```python
from build123d import *

# Parameters (mm, degrees)
BOSS_EXTRUDE1_DEPTH = 1.5875
SKETCH3_R           = 2.032
SKETCH3_R_2         = 1.778
CUT_EXTRUDE1_DEPTH  = 52.085937461
CUT_EXTRUDE2_DEPTH  = 52.085937461
FILLET1_R           = 6.35
FILLET2_R           = 1.5875


with BuildPart() as part:
    # Sketch1 → Boss-Extrude1 (new body)
    with BuildSketch(Plane(origin=(0, 0, 0), x_dir=(1, 0, 0), z_dir=(0, 1, 0))):
        with BuildLine():
            Line((0, 0), (18.415, -19.05))
            Line((18.415, -19.05), (18.415, -47.625))
            ThreePointArc((18.415, -47.625), (0, -46.266231115), (-18.415, -47.625))
            Line((-18.415, -47.625), (-18.415, -19.05))
            Line((-18.415, -19.05), (0, 0))
        make_face()
    extrude(amount=BOSS_EXTRUDE1_DEPTH)

    # Sketch3 → Cut-Extrude1 (cut, through all)
    with BuildSketch(Plane(origin=(0, 1.5875, 0), x_dir=(1, 0, 0), z_dir=(0, 1, 0))):
        with Locations(Location((12.7, -42.294109534, 0), (0, 0, 270))):
            Circle(SKETCH3_R)
        with Locations(Location((-12.7, -42.294109534, 0), (0, 0, 270))):
            Circle(SKETCH3_R)
        with Locations(Location((-12.7, -23.244109534, 0), (0, 0, 270))):
            Circle(SKETCH3_R)
        with Locations(Location((12.7, -23.244109534, 0), (0, 0, 270))):
            Circle(SKETCH3_R_2)
        with Locations(Location((0, -7.9375, 0), (0, 0, 270))):
            Circle(SKETCH3_R)
    extrude(amount=-CUT_EXTRUDE1_DEPTH, mode=Mode.SUBTRACT)

    # Sketch4 → Cut-Extrude2 (cut, through all)
    with BuildSketch(Plane(origin=(0, 1.5875, 0), x_dir=(1, 0, 0), z_dir=(0, 1, 0))):
        with BuildLine():
            Line((7.9375, -36.974796609), (7.9375, -23.286267168))
            Line((7.9375, -23.286267168), (0, -15.075060272))
            Line((0, -15.075060272), (-7.9375, -23.286267168))
            Line((-7.9375, -23.286267168), (-7.9375, -36.974796609))
            ThreePointArc((-7.9375, -36.974796609), (0, -36.741231115), (7.9375, -36.974796609))
        make_face()
    extrude(amount=-CUT_EXTRUDE2_DEPTH, mode=Mode.SUBTRACT)

    # Fillet1
    fillet1_edges = [part.edges().sort_by_distance(p)[0] for p in [
        (0, 0.79375, 0),
        (18.415, 0.79375, 19.05),
        (18.415, 0.79375, 47.625),
        (-18.415, 0.79375, 47.625),
        (-18.415, 0.79375, 19.05),
    ]]
    fillet(fillet1_edges, radius=FILLET1_R)

    # Fillet2
    fillet2_edges = [part.edges().sort_by_distance(p)[0] for p in [
        (-7.9375, 0.79375, 23.286267168),
        (0, 0.79375, 15.075060272),
        (7.9375, 0.79375, 23.286267168),
        (7.9375, 0.79375, 36.974796609),
        (-7.9375, 0.79375, 36.974796609),
    ]]
    fillet(fillet2_edges, radius=FILLET2_R)


solid = part.part
```
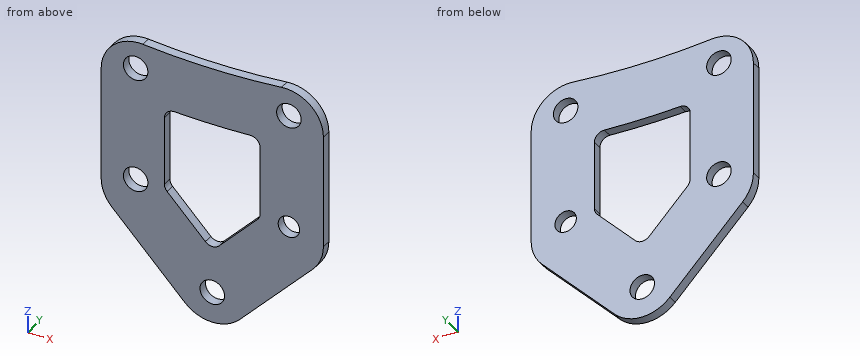
The listing builds one solid part. Answer for the finished solid, in the listing's coordinates (mm). Round coordinates to 2 decimals unless told otherwise and drop trailing zeros. Loops run counter-clockwise (first coordinate to the right, second up) from the corner with the lowest first, then second, coordinate; pieces in that order, holes last. Notation, with made-up numbers: (-31, 44.5) - (3, 44.5) arc R21 ccw to (3, 66.5) - close; hole circle Ø7 at (28, 52.5). An arc over 180 degrees is marked (long way). Use one line per item in the form item = value. Start each with the question number.
1. The part is cut by section B-B on y = 1. Give the number of separate pieces and of enclosed holes in the cut face, then the cut area to 3 significant figures.
2. The part is cut by section C-C on z = 28.5. Determine the outline of the cut face in (x, y) (1 decimal), then the cut area to 3 significant figures.
3. The part is cut by section D-D on x = -5.5. Determine the outline of the cut face in (y, z), then the cut area to 3 significant figures.
4. Consider line 1 (X direction, y = 1.35, z = 28.5) (1 decimal); line 2 (X direction, y = 1.05, z = 43.5); line 3 (X direction, y = 0.9, z = 24) (1 decimal). Determine where each line is inside the solid, lowest interval first. Write a range as [from, to].
5. The part is cut by section A-A on x = 0. Determine the outline of the cut face in (y, z).
Geometry check:
q1.separate_pieces = 1
q1.enclosed_holes = 6
q1.area = 997 mm^2
q2.outline = (-18.4, 0) - (-7.9, 0) - (-7.9, 1.6) - (-18.4, 1.6) - close; (7.9, 0) - (18.4, 0) - (18.4, 1.6) - (7.9, 1.6) - close
q2.area = 33.3 mm^2
q3.outline = (0, 5.69) - (1.59, 5.69) - (1.59, 20.76) - (0, 20.76) - close; (0, 36.85) - (1.59, 36.85) - (1.59, 46.39) - (0, 46.39) - close
q3.area = 39.1 mm^2
q4.line_1 = [-18.4, -7.9], [7.9, 18.4]
q4.line_2 = [-17.65, -14.34], [-11.06, 11.06], [14.34, 17.65]
q4.line_3 = [-18.4, -14.6], [-10.8, -7.9], [7.9, 11.1], [14.3, 18.4]
q5.outline = (0, 2.79) - (1.59, 2.79) - (1.59, 5.91) - (0, 5.91) - close; (0, 9.97) - (1.59, 9.97) - (1.59, 15.77) - (0, 15.77) - close; (0, 36.74) - (1.59, 36.74) - (1.59, 46.27) - (0, 46.27) - close
